Can you work these out from the model? Positions are in its coordinate system, mm. A direction names the side the tool comes from. Give positions to 0.01 mm unless a question says otherwise; leave off trailing zeros. Loops run counter-clockwise (first coordinate to the right, second up) from the corner with the lowest first, then second, coordinate; pieces in that order, holes last. Notation, with made-up numbers: M 9,-12 L 48,-12 A12 cw 48,7 Z; hole C 59,25.5 d10. An arc over 180 degrees is marked long. Answer as a JSON object with one key per item and string values.
```python
from build123d import *

# Parameters (mm, degrees)
SKETCH1_R           = 55
SKETCH1_R_2         = 35
BOSS_EXTRUDE1_DEPTH = 5
SKETCH2_W           = 5
SKETCH2_H           = 10
CUT_EXTRUDE1_DEPTH  = 5


with BuildPart() as part:
    # Sketch1 → Boss-Extrude1 (new body)
    with BuildSketch(Plane(origin=(0, 0, 0), x_dir=(1, 0, 0), z_dir=(0, 1, 0))):
        with Locations(Location((0, 0, 0), (0, 0, 270))):
            Circle(SKETCH1_R)
        with Locations(Location((0, 0, 0), (0, 0, 270))):
            Circle(SKETCH1_R_2, mode=Mode.SUBTRACT)
    extrude(amount=BOSS_EXTRUDE1_DEPTH)

    # Sketch2 → Cut-Extrude1 (cut)
    with BuildSketch(Plane(origin=(0, 5, 0), x_dir=(1, 0, 0), z_dir=(0, 1, 0))):
        with Locations((-42.5, 0)):
            Rectangle(SKETCH2_W, SKETCH2_H)
        with Locations((47.5, 0)):
            Rectangle(SKETCH2_W, SKETCH2_H)
    extrude(amount=-CUT_EXTRUDE1_DEPTH, mode=Mode.SUBTRACT)


solid = part.part
```
1) If we mould it in two halves opening along X, with no side actions, what happens to faces 3 (the flat face through (-43, 3, -5)), 4 (the cylindrical face through (-48.794, 2.465, 25.379)), 5 (the flat face through (-36, 0, -1))? For each: +X half, -X half, draft (parallel to the pull), parting line (faces both ways), or undercut.
Answer list:
{"face 3": "undercut", "face 4": "parting line", "face 5": "draft"}
2) Suppose I cut it at A-A, the plane x = 0. Write out the boundary of the cut face in (y, z).
Answer list:
{"outline": "M 0,-55 L 5,-55 L 5,-35 L 0,-35 Z; M 0,35 L 5,35 L 5,55 L 0,55 Z"}
3) Suppose I cut it at B-B, the plane z = 0. Write out the boundary of the cut face in (x, y).
Answer list:
{"outline": "M -55,0 L -45,0 L -45,5 L -55,5 Z; M -40,0 L -35,0 L -35,5 L -40,5 Z; M 35,0 L 45,0 L 45,5 L 35,5 Z; M 50,0 L 55,0 L 55,5 L 50,5 Z"}
4) Will these pins go through, and if not, where does the flat tip stop? pin 1 Ø3 at (y, z) = (3.5, 19.5) entering from +X; pin 2 Ø1.5 at (x, y) = (-43, 1.5) entering from +Z; pin 3 Ø1.5 at (y, z) = (2.5, 1) entering from -X.
Answer list:
{"pin 1": "x = 51.97", "pin 2": "z = 35.21", "pin 3": "x = -55"}
5) For faces 1 (the flat face through (47, 3, 5)), 2 (the flat face through (-36, 5, -1)), which set-ups out of +Z, -Z, +X, -X, +Y, -Y let a thin tool reach every point of the face, with its end or its side?
Answer list:
{"face 1": "+Y, -Y", "face 2": "+Z, -Z, +X, -X, +Y"}
6) Please list where these lines run through material, in increasing order: line 1 along X through (y, z) = (2.5, 0); line 2 along Z through (x, y) = (30.5, 1.1); line 3 along Z through (x, y) = (-20, 0.65). Write a range as from..to.
Answer list:
{"line 1": "-55..-45, -40..-35, 35..45, 50..55", "line 2": "-45.77..-17.17, 17.17..45.77", "line 3": "-51.23..-28.72, 28.72..51.23"}
7) Suppose I cut it at D-D, the plane z = 14. Write out the boundary of the cut face in (x, y), and give its area (3 significant figures).
Answer list:
{"outline": "M -53.19,0 L -32.08,0 L -32.08,5 L -53.19,5 Z; M 32.08,0 L 53.19,0 L 53.19,5 L 32.08,5 Z", "area": "211 mm^2"}
8) Suppose I cut it at C-C, the plane y = 2.95. Write out the boundary of the cut face in (x, z), and give its area (3 significant figures).
Answer list:
{"outline": "C 0,0 d110; hole M -45,-5 L -40,-5 L -40,5 L -45,5 Z; hole C 0,0 d70; hole M 45,-5 L 50,-5 L 50,5 L 45,5 Z", "area": "5,550 mm^2"}
